The listing builds one solid part. Answer for the finished solid, in the listing's coordinates (mm). A direction names the side the tool comes from. Round coordinates to 2 decimals unless told otherwise and drop trailing zeros. Write each loop counter-clockwise with the first axis right and the second up, starting at its lowest first coordinate (ties: lowest second). Pieces come first, ordered by that corner, then holes. Notation, with made-up numbers: (87.25, -9) - (97.25, -9) arc R37 cw to (97.25, 29) - close; hole circle Ø6 at (-19, 12.5). An arc over 180 degrees is marked (long way). Return JSON: item names as keys, results as strings. Group by question number.
(1) Which of the six approach directions +Z, -Z, +X, -X, +Y, -Y give full straight-line access (tool end or side, diameter ignored) to faces 4 (the cylindrical face through (-35.833, 9.86, -19.751)), 5 (the flat face through (5, 31, -36)), 6 (the cylindrical face through (0, 40, 30))?
(2) Section D-D, the plane z = -22 is taken. Write down the section's boundary in (x, y), then the cut area to 3 significant figures.
(3) Each of these flat-tipped pins is pushed along its axis until it touches: pin 1 (12 mm diameter, centred on x = 51.5, y = 7, fed in from -Z); pin 2 (8 mm diameter, centred on y = 14, z = -76.5, fed in from +X); pin 3 (10 mm diameter, centred on y = 18, z = -53, fed in from +X); pin 4 (1 mm diameter, centred on x = 47.5, y = 26, fed in from +Z). Where does it stop, or does it pass through?
(4) Section A-A, the plane y = 17 is taken. Write down the section's boundary in (x, z), then the cut area to 3 significant figures.
(5) Section B-B, the plane x = 0 is taken. Write down the section's boundary in (y, z).
(6) Section C-C, the plane z = 3.5 is taken. Write down the section's boundary in (x, y), then the cut area to 3 significant figures.
(7) Find the intervals of material crossed by line 1 along X through (y, z) = (40.5, 0); line 2 along Z through (x, y) = (0, 19); line 3 along Z through (x, y) = (0, 35), in increasing order. Write a range as [from, to].
(8) Determine the mould class of faces 1 (the cylindrical face through (-0.176, 10.14, -58.502)), 2 (the flat face through (-19, 0, 4)), 3 (the flat face through (-68.256, 10.14, 30.17)) for opening direction Z: +Z half, -Z half, draft (parallel to the pull), parting line (faces both ways), or undercut.
```python
from build123d import *

# Parameters (mm, degrees)
SKETCH1_R           = 82.5
SKETCH1_R_2         = 30
BOSS_EXTRUDE2_DEPTH = 20
SKETCH1_4_R         = 30
SKETCH1_4_R_2       = 17.5
BOSS_EXTRUDE3_DEPTH = 60
SKETCH3_W           = 50
SKETCH3_H           = 40
BOSS_EXTRUDE4_DEPTH = 5
CIRPATTERN1_COUNT   = 3
CUT_EXTRUDE5_DEPTH  = 10
CIRPATTERN4_COUNT   = 3
CUT_EXTRUDE7_DEPTH  = 21
CIRPATTERN5_COUNT   = 3
CUT_EXTRUDE8_DEPTH  = 21
FILLET1_R           = 20


with BuildPart() as part:
    # Sketch1 → Boss-Extrude2 (new body)
    with BuildSketch(Plane(origin=(0, 0, 0), x_dir=(1, 0, 0), z_dir=(0, 1, 0))):
        Circle(SKETCH1_R)
        Circle(SKETCH1_R_2, mode=Mode.SUBTRACT)
    extrude(amount=BOSS_EXTRUDE2_DEPTH)

    # Sketch1_4 → Boss-Extrude3 (add)
    with BuildSketch(Plane(origin=(0, 0, 0), x_dir=(1, 0, 0), z_dir=(0, 1, 0))):
        Circle(SKETCH1_4_R)
        Circle(SKETCH1_4_R_2, mode=Mode.SUBTRACT)
    extrude(amount=BOSS_EXTRUDE3_DEPTH)

    # Sketch3 → Boss-Extrude4 (add, symmetric)
    with BuildSketch(Plane(origin=(0, 0, 0), x_dir=(0, 0, -1), z_dir=(1, 0, 0))):
        with Locations((42.5, 40)):
            Rectangle(SKETCH3_W, SKETCH3_H)
    boss_extrude4 = extrude(amount=BOSS_EXTRUDE4_DEPTH, both=True)

    # CirPattern1: Boss-Extrude4 ×3 about axis
    cirpattern1_axis = Axis((0, 0, 0), (0, 1, 0))
    for i in range(1, CIRPATTERN1_COUNT):
        add(boss_extrude4.rotate(cirpattern1_axis, i * 360 / CIRPATTERN1_COUNT))

    # Sketch15 → Cut-Extrude5 (cut)
    with BuildSketch(Plane(origin=(5, 0, 0), x_dir=(0, 0, -1), z_dir=(1, 0, 0))):
        Polygon((29.580398915, 60), (54.580398915, 20), (67.5, 20), (67.5, 60), align=None)
    cut_extrude5 = extrude(amount=-CUT_EXTRUDE5_DEPTH, mode=Mode.SUBTRACT)

    # CirPattern4: Cut-Extrude5 ×3 about axis
    cirpattern4_axis = Axis((0, 0, 0), (0, 1, 0))
    for i in range(1, CIRPATTERN4_COUNT):
        add(cut_extrude5.rotate(cirpattern4_axis, i * 360 / CIRPATTERN4_COUNT), mode=Mode.SUBTRACT)

    # Sketch22 → Cut-Extrude7 (cut, through all)
    with BuildSketch(Plane(origin=(0, 20, 0), x_dir=(1, 0, 0), z_dir=(0, 1, 0))):
        with BuildLine():
            Line((8, 66.5), (8, 82.111205082))
            ThreePointArc((8, 82.111205082), (0, 82.5), (-8, 82.111205082))
            Line((-8, 82.111205082), (-8, 66.5))
            ThreePointArc((-8, 66.5), (0, 58.5), (8, 66.5))
        make_face()
    cut_extrude7 = extrude(amount=-CUT_EXTRUDE7_DEPTH, mode=Mode.SUBTRACT)

    # CirPattern5: Cut-Extrude7 ×3 about axis
    cirpattern5_axis = Axis((0, 0, 0), (0, 1, 0))
    for i in range(1, CIRPATTERN5_COUNT):
        add(cut_extrude7.rotate(cirpattern5_axis, i * 360 / CIRPATTERN5_COUNT), mode=Mode.SUBTRACT)

    # Sketch29 → Cut-Extrude8 (cut, through all)
    with BuildSketch(Plane(origin=(0, 20, 0), x_dir=(1, 0, 0), z_dir=(0, 1, 0))):
        with BuildLine():
            Line((-80.510468766, -18.008731746), (-34.681233917, 18.959795028))
            Line((-34.681233917, 18.959795028), (-24.659817795, 78.728288349))
            ThreePointArc((-24.659817795, 78.728288349), (-71.447253677, 41.249726568), (-80.510468766, -18.008731746))
        make_face()
        with BuildLine():
            Line((24.659817795, 78.728288349), (34.681233917, 18.959795028))
            Line((34.681233917, 18.959795028), (80.510468766, -18.008731746))
            ThreePointArc((80.510468766, -18.008731746), (71.447253677, 41.249726568), (24.659817795, 78.728288349))
        make_face()
        with BuildLine():
            Line((-55.850650713, -60.720299859), (0, -39.52545779))
            Line((0, -39.52545779), (55.850650713, -60.720299859))
            ThreePointArc((55.850650713, -60.720299859), (0, -82.5), (-55.850650713, -60.720299859))
        make_face()
    extrude(amount=-CUT_EXTRUDE8_DEPTH, mode=Mode.SUBTRACT)

    # Fillet1
    fillet1_edges = [part.edges().sort_by_distance(p)[0] for p in [
        (0, 10, 39.52545779),
        (34.681233917, 10, -18.959795028),
        (-34.681233917, 10, -18.959795028),
    ]]
    fillet(fillet1_edges, radius=FILLET1_R)


solid = part.part
```
Working result:
{
 "1": {"face 4": "-Z, -X, +Y, -Y", "face 5": "-Z, +X, +Y", "face 6": "+Z, +Y"},
 "2": {"outline": "(-34.72, 0) - (34.72, 0) - (34.72, 20) - (20.4, 20) - (20.4, 60) - (-20.4, 60) - (-20.4, 20) - (-34.72, 20) - close", "area": "3,020 mm^2"},
 "3": {"pin 1": "stops at z = -10.23", "pin 2": "stops at x = 25.7", "pin 3": "stops at x = 29.81", "pin 4": "passes through"},
 "4": {"outline": "(-80.51, 18.01) - (-40.59, -14.19) arc R20 cw to (-33.43, -26.45) - (-24.66, -78.73) arc R82.5 ccw to (-8, -82.11) - (-8, -66.5) arc R8 cw to (8, -66.5) - (8, -82.11) arc R82.5 ccw to (24.66, -78.73) - (33.43, -26.45) arc R20 cw to (40.59, -14.19) - (80.51, 18.01) arc R82.5 ccw to (75.11, 34.13) - (61.59, 26.32) arc R8 cw to (53.59, 40.18) - (67.11, 47.98) arc R82.5 ccw to (55.85, 60.72) - (7.1, 42.22) arc R20 cw to (-7.1, 42.22) - (-55.85, 60.72) arc R82.5 ccw to (-67.11, 47.98) - (-53.59, 40.18) arc R8 cw to (-61.59, 26.32) - (-75.11, 34.13) arc R82.5 ccw to start; hole circle Ø35 at (0, 0)", "area": "10,800 mm^2"},
 "5": {"outline": "(0, -58.5) - (20, -58.5) - (20, -54.58) - (60, -29.58) - (60, -17.5) - (0, -17.5) - close; (0, 17.5) - (60, 17.5) - (60, 30) - (20, 30) - (20, 40.92) - (0, 40.92) - close"},
 "6": {"outline": "(-62.52, 0) - (-17.15, 0) - (-17.15, 60) - (-29.8, 60) - (-29.8, 20) - (-62.52, 20) - close; (17.15, 0) - (62.52, 0) - (62.52, 20) - (29.8, 20) - (29.8, 60) - (17.15, 60) - close", "area": "2,830 mm^2"},
 "7": {"line 1": "x = [-30, -17.5], [17.5, 30]", "line 2": "z = [-58.5, -17.5], [17.5, 40.92]", "line 3": "z = [-45.21, -17.5], [17.5, 30]"},
 "8": {"face 1": "-Z half", "face 2": "draft", "face 3": "undercut"}
}
